Source: CAD feature listing. Evaluate the final solid. Frame: model axes, mm. A direction names the side the tool comes from. Round coordinates to 2 decimals unless told otherwise and drop trailing zeros. Loops run counter-clockwise (first coordinate to the right, second up) from the corner with the lowest first, then second, coordinate; pieces in that order, holes last. Notation, with made-up numbers: (55.25, -6) - (63.25, -6) arc R19 cw to (63.25, 25) - close; hole circle Ø2 at (74.25, 89.5). An arc over 180 degrees is marked (long way). One line per question, with ' | ' between items. Start each with the question number.
1. Cut plane C-C (x = -0.5). Return loops of the section in (y, z).
2. Ray query, line 1 (Y direction, x = -3.5, z = 3.7); line 2 (X direction, y = -2.5, z = 3.5); line 3 (X direction, y = 13.5, z = 0.8). Return the intervals inside material, ascending.
3. Cut plane A-A (z = 1.75). Return loops of the section in (x, y), then the cut area to 3 significant figures.
4. Access query for faces 1 (the flat face through (12, -3, 3)), 2 (the flat face through (-3, 18.75, 3)). Directions: +Z, -Z, +X, -X, +Y, -Y. A direction counts if a zero-diameter tool reaches every point of the face in a straight line with its end or side. Return the directions, or none.
5. Pin query (flat end, axial travel): pin 1 (1 mm diameter, centred on x = 14.5, z = 1.5, fed in from +Y); pin 2 (4 mm diameter, centred on x = -0.5, y = 13.5, fed in from -Z); pin 3 (1.5 mm diameter, centred on x = 9, y = -1.5, fed in from -Z); pin 4 (1.8 mm diameter, centred on y = 3, z = 2.5, fed in from -X). Return the tip coordinate at first contact, or that it passes through.
6. Cut plane B-B (y = 15). Return loops of the section in (x, z), then the cut area to 3 significant figures.
```python
from build123d import *

# Parameters (mm, degrees)
BOSS_EXTRUDE1_DEPTH = 6


with BuildPart() as part:
    # Sketch1 → Boss-Extrude1 (new body)
    with BuildSketch(Plane.XY):
        Polygon((0, 0), (0, 8.75), (-6, 8.75), (-6, 18.75), (0, 18.75), (17, 0), (17, -6), (12, -6), (12, 0), align=None)
    extrude(amount=BOSS_EXTRUDE1_DEPTH)


solid = part.part
```
Answers follow:
1) outline: (8.75, 0) - (18.75, 0) - (18.75, 6) - (8.75, 6) - close
2) line 1: y = 8.75 to 18.75 | line 2: x = 12 to 17 | line 3: x = -6 to 4.76
3) outline: (-6, 8.75) - (0, 8.75) - (0, 0) - (12, 0) - (12, -6) - (17, -6) - (17, 0) - (0, 18.75) - (-6, 18.75) - close | area: 249 mm2
4) face 1: +Z, -Z, -X, -Y | face 2: +Z, -Z, +X, -X, +Y
5) pin 1: stops at y = 3.31 | pin 2: stops at z = 0 | pin 3: passes through | pin 4: stops at x = 0
6) outline: (-6, 0) - (3.4, 0) - (3.4, 6) - (-6, 6) - close | area: 56.4 mm2
